Geometry check sheet. Reference: the model listing, model coordinates, mm. A direction names the side the tool comes from. Give positions to 0.01 mm unless a question says otherwise; leave off trailing zeros. Loops run counter-clockwise (first coordinate to the right, second up) from the corner with the lowest first, then second, coordinate; pieces in that order, holes last. Notation, with made-up numbers: (-17.75, 67) -> (6.25, 67) arc R23 ccw to (6.25, 100) -> close; hole circle Ø7 at (46, 42). An arc over 180 degrees is marked (long way). Write each question's results on one line, items separated by ' | '. Start each with the question number.
1) Sectioned sample at A-A on x = 3.81. Record the cut outline in (y, z).
2) Draft check along X on faces 3 (the face through (12, 19.516, -2)), 4 (the face through (0, 8, 13)), 5 (the face through (18.064, -6.455, -1.665)). Enter one of: pulls with the +X half, pulls with the -X half, needs draft (parallel to the pull), parting line crosses it, or undercut.
3) Set-up check for faces 1 (the face through (12, 8, 9.757)), 2 (the face through (12, 8, -18.718)): record each of +Z, -Z, +X, -X, +Y, -Y from which the full face is reachable in a straight line by a thin tool's end or side.
4) Sectioned sample at D-D on x = 12.5. Record the cut outline in (y, z).
5) Sectioned sample at B-B on y = 18.5. Record the cut outline in (x, z), then the cut area to 3 significant figures.
6) Sectioned sample at C-C on z = -10.5. Record the cut outline in (x, y).
7) Scan lines: line 1 (Z direction, x = 8.5, y = 14); line 2 (Y direction, x = 17.75, z = -12.5); line 3 (X direction, y = 23.5, z = -1). Record each from-to range of solid material in increasing order. Write a range as from..to.
```python
from build123d import *

# Parameters (mm, degrees)
SKETCH1_W           = 33.554975054
SKETCH1_H           = 33.554975054
SKETCH1_W_2         = 23.394975054
SKETCH1_H_2         = 23.394975054
BOSS_EXTRUDE1_DEPTH = 23.837801194
SKETCH2_R           = 1.27
CUT_EXTRUDE1_DEPTH  = 46.216489821


with BuildPart() as part:
    # Sketch1 → Boss-Extrude1 (new body)
    with BuildSketch(Plane(origin=(0, 0, 0), x_dir=(0, 0, -1), z_dir=(1, 0, 0))):
        with Locations((1.94025366, 7.818080922)):
            Rectangle(SKETCH1_W, SKETCH1_H)
        with Locations((1.94025366, 7.818080922)):
            Rectangle(SKETCH1_W_2, SKETCH1_H_2, mode=Mode.SUBTRACT)
    extrude(amount=BOSS_EXTRUDE1_DEPTH)

    # Sketch2 → Cut-Extrude1 (cut, through all)
    with BuildSketch(Plane.XZ.offset(8.959406605)):
        with Locations(Location((3.81, -1.94025366, 0), (0, 0, 270))):
            Circle(SKETCH2_R)
        with Locations(Location((19.304, -1.94025366, 0), (0, 0, 270))):
            Circle(SKETCH2_R)
    extrude(amount=-CUT_EXTRUDE1_DEPTH, mode=Mode.SUBTRACT)


solid = part.part
```
Result:
1) outline: (-8.96, -18.72) -> (24.6, -18.72) -> (24.6, -3.21) -> (19.52, -3.21) -> (19.52, -13.64) -> (-3.88, -13.64) -> (-3.88, -3.21) -> (-8.96, -3.21) -> close; (-8.96, -0.67) -> (-3.88, -0.67) -> (-3.88, 9.76) -> (19.52, 9.76) -> (19.52, -0.67) -> (24.6, -0.67) -> (24.6, 14.84) -> (-8.96, 14.84) -> close
2) face 3: needs draft | face 4: pulls with the -X half | face 5: undercut
3) face 1: +X, -X | face 2: -Z, +X, -X, +Y, -Y
4) outline: (-8.96, -18.72) -> (24.6, -18.72) -> (24.6, 14.84) -> (-8.96, 14.84) -> close; hole (-3.88, -13.64) -> (19.52, -13.64) -> (19.52, 9.76) -> (-3.88, 9.76) -> close
5) outline: (0, -18.72) -> (23.84, -18.72) -> (23.84, -13.64) -> (0, -13.64) -> close; (0, 9.76) -> (23.84, 9.76) -> (23.84, 14.84) -> (0, 14.84) -> close | area: 242 mm^2
6) outline: (0, -8.96) -> (23.84, -8.96) -> (23.84, -3.88) -> (0, -3.88) -> close; (0, 19.52) -> (23.84, 19.52) -> (23.84, 24.6) -> (0, 24.6) -> close
7) line 1: -18.72..-13.64, 9.76..14.84 | line 2: -8.96..-3.88, 19.52..24.6 | line 3: 0..2.96, 4.66..18.45, 20.16..23.84
